Geometry check sheet. Reference: drawing and pictorial views, mm from the part's lowest x, y, z. Coordinates: 2 decimals unless noted, no trailing zeros. Loops run counter-clockwise (first coordinate to the right, second up) from the corner with the lowest first, then second, coordinate; pieces in that order, holes last. Notation, with made-up numbers: (86, -1) -> (135, -1) arc R17 cw to (135, 15) -> close; hole circle Ø3 at (5.25, 42.5). An arc over 180 degrees is marked (long way). Answer as a JSON object with one key per item and string values.
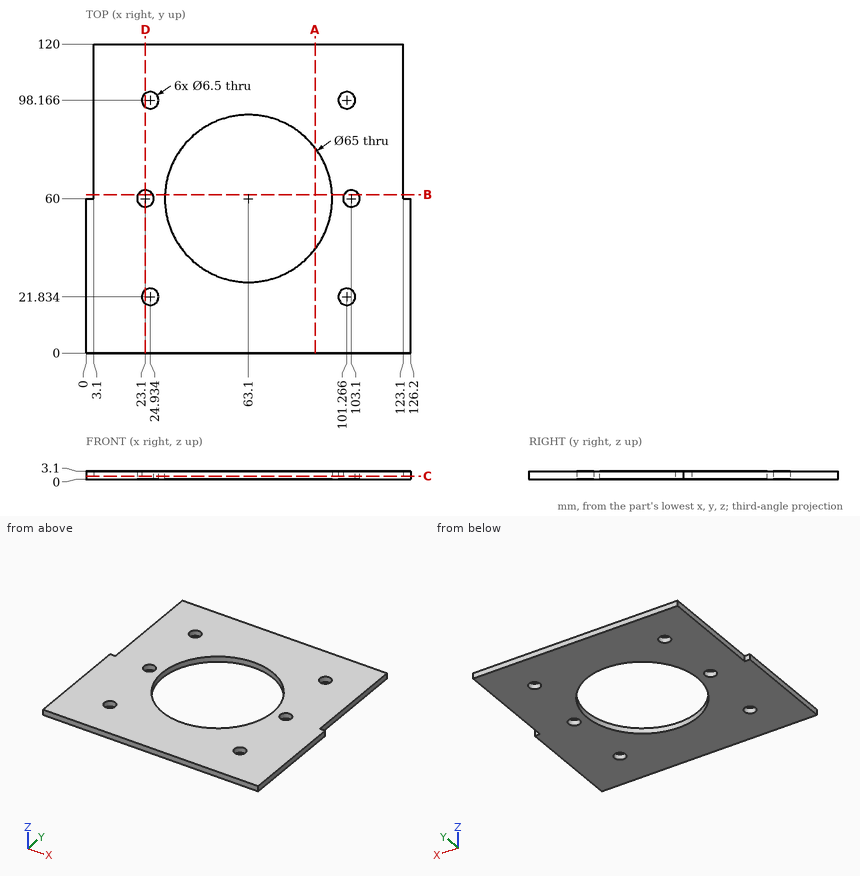
1. Section check C-C, the plane z = 1.15. Record the boundary of the cut face in (x, y), then the cut area to 3 significant figures.
Evaluation:
{"outline": "(0, 0) -> (126.2, 0) -> (126.2, 60) -> (123.1, 60) -> (123.1, 120) -> (3.1, 120) -> (3.1, 60) -> (0, 60) -> close; hole circle Ø6.5 at (23.1, 60); hole circle Ø6.5 at (24.93, 21.83); hole circle Ø6.5 at (24.93, 98.17); hole circle Ø65 at (63.1, 60); hole circle Ø6.5 at (101.27, 21.83); hole circle Ø6.5 at (101.27, 98.17); hole circle Ø6.5 at (103.1, 60)", "area": "11,300 mm^2"}
2. Section check A-A, the plane x = 89. Record the boundary of the cut face in (y, z).
Evaluation:
{"outline": "(0, 0) -> (40.37, 0) -> (40.37, 3.1) -> (0, 3.1) -> close; (79.63, 0) -> (120, 0) -> (120, 3.1) -> (79.63, 3.1) -> close"}
3. Thickness scan on probe 1 along Y at (x, z) = (102, 1.35); probe 2 along X at (y, z) = (96, 2.1); probe 3 along Y at (x, z) = (62.5, 0.9). Record the ranges inside material, lowest first. Write a range as from..to.
Evaluation:
{"probe 1": "y = 0..18.67, 25..56.94, 63.06..95, 101.33..120", "probe 2": "x = 3.1..22.51, 27.36..98.84, 103.69..123.1", "probe 3": "y = 0..27.51, 92.49..120"}
4. Section check D-D, the plane x = 23.1. Record the boundary of the cut face in (y, z).
Evaluation:
{"outline": "(0, 0) -> (19.15, 0) -> (19.15, 3.1) -> (0, 3.1) -> close; (24.52, 0) -> (56.75, 0) -> (56.75, 3.1) -> (24.52, 3.1) -> close; (63.25, 0) -> (95.48, 0) -> (95.48, 3.1) -> (63.25, 3.1) -> close; (100.85, 0) -> (120, 0) -> (120, 3.1) -> (100.85, 3.1) -> close"}
5. Section check B-B, the plane y = 61.5. Record the boundary of the cut face in (x, z), then the cut area to 3 significant figures.
Evaluation:
{"outline": "(3.1, 0) -> (20.22, 0) -> (20.22, 3.1) -> (3.1, 3.1) -> close; (25.98, 0) -> (30.63, 0) -> (30.63, 3.1) -> (25.98, 3.1) -> close; (95.57, 0) -> (100.22, 0) -> (100.22, 3.1) -> (95.57, 3.1) -> close; (105.98, 0) -> (123.1, 0) -> (123.1, 3.1) -> (105.98, 3.1) -> close", "area": "135 mm^2"}
6. Depth check by flat-ended pin: P1, Ø0.9, axis at x = 2, z = 1, coming from the +Y side; P2, Ø10, axis at x = 107, y = 22, coming from the -Z side; P3, Ø1.5, axis at y = 85, z = 1, coming from the +X side; P4, Ø1.5, axis at y = 101, z = 1, coming from the -X side. Enter the tip coordinate at first touch or a pass-through.
Evaluation:
{"P1": "stops at y = 60", "P2": "stops at z = 0", "P3": "stops at x = 123.1", "P4": "stops at x = 3.1"}
